from build123d import *

# Parameters (mm, degrees)
SKETCH1_W           = 127
SKETCH1_H           = 127
BOSS_EXTRUDE1_DEPTH = 127
SKETCH2_W           = 96.52
SKETCH2_H           = 96.52
CUT_EXTRUDE1_DEPTH  = 118.11
SKETCH3_W           = 101.6
SKETCH3_H           = 101.6
SKETCH3_W_2         = 96.52
SKETCH3_H_2         = 96.52
CUT_EXTRUDE2_DEPTH  = 6.35
SKETCH5_W           = 96.52
SKETCH5_H           = 105.41
CUT_EXTRUDE3_DEPTH  = 6.35
SKETCH6_W           = 109.22
SKETCH6_H           = 105.41
CUT_EXTRUDE4_DEPTH  = 6.35


with BuildPart() as part:
    # Sketch1 → Boss-Extrude1 (new body)
    with BuildSketch(Plane.XY):
        Rectangle(SKETCH1_W, SKETCH1_H)
    extrude(amount=BOSS_EXTRUDE1_DEPTH)

    # Sketch2 → Cut-Extrude1 (cut)
    with BuildSketch(Plane(origin=(0, 63.5, 0), x_dir=(1, 0, 0), z_dir=(0, 1, 0))):
        with Locations((0, -63.5)):
            Rectangle(SKETCH2_W, SKETCH2_H)
    extrude(amount=-CUT_EXTRUDE1_DEPTH, mode=Mode.SUBTRACT)

    # Sketch3 → Cut-Extrude2 (cut)
    with BuildSketch(Plane(origin=(0, 63.5, 0), x_dir=(1, 0, 0), z_dir=(0, 1, 0))):
        with Locations((0, -63.5)):
            Rectangle(SKETCH3_W, SKETCH3_H)
        with Locations((0, -63.5)):
            Rectangle(SKETCH3_W_2, SKETCH3_H_2, mode=Mode.SUBTRACT)
    extrude(amount=-CUT_EXTRUDE2_DEPTH, mode=Mode.SUBTRACT)

    # Sketch5 → Cut-Extrude3 (cut)
    with BuildSketch(Plane.XY.offset(15.24)):
        with Locations((0, -1.905)):
            Rectangle(SKETCH5_W, SKETCH5_H)
    cut_extrude3 = extrude(amount=-CUT_EXTRUDE3_DEPTH, mode=Mode.SUBTRACT)

    # Mirror1: Cut-Extrude3 across plane
    add(cut_extrude3.mirror(Plane(origin=(0, 0, 63.5), x_dir=(1, 0, 0), z_dir=(0, 0, -1))), mode=Mode.SUBTRACT)

    # Sketch6 → Cut-Extrude4 (cut)
    with BuildSketch(Plane.ZY.offset(-48.26)):
        with Locations((63.5, -1.905)):
            Rectangle(SKETCH6_W, SKETCH6_H)
    cut_extrude4 = extrude(amount=-CUT_EXTRUDE4_DEPTH, mode=Mode.SUBTRACT)

    # Mirror2: Cut-Extrude4 across plane
    add(cut_extrude4.mirror(Plane(origin=(0, 0, 0), x_dir=(0, 0, 1), z_dir=(1, 0, 0))), mode=Mode.SUBTRACT)


solid = part.part
Model file for the job. Use its own axes, mm. A direction names the side the tool comes from. Coordinates: 2 decimals unless noted, no trailing zeros. Write each loop counter-clockwise with the first axis right and the second up, starting at its lowest first coordinate (ties: lowest second). Pieces come first, ordered by that corner, then holes. Notation, with made-up numbers: (4, 78) -> (44, 78) arc R9 ccw to (44, 92) -> close; hole circle Ø10 at (-31.75, 28.25). An arc over 180 degrees is marked (long way). One line per item, written item: value. Start each with the question number.
1) Slice it at C-C on z = 93.5. Write the cut outline in (x, y).
2) Probe probe 1 along Y at (x, z) = (52.5, 93); probe 2 along X at (y, z) = (-3, 11); probe 3 along Z at (x, y) = (-53.5, 0). List the from-to ranges inside material, lowest first.
3) Slice it at B-B on x = -7. Write the cut outline in (y, z).
4) Slice it at A-A on y = -6. Write the cut outline in (x, z), then the cut area to 3 significant figures.
5) Which spindle directions (+Z, -Z, +X, -X, +Y, -Y) get a long thin tool onto all of the face, cutting with end or side? Do faces 1 (the face through (-63.5, -1, 63)), 2 (the face through (-49, 50.8, 63)), 3 (the face through (-1, 54, 15.24)). Say none if no direction does.
6) Pull direction Z, two halves, no side cores. Call faces 4 (the face through (-1, -63.5, 63)), 5 (the face through (-1, 1, 127)), 6 (the face through (-1, -1, 118.11)), 7 (the face through (-1, 1, 0)): +Z half, -Z half, draft (parallel to the pull), parting line (faces both ways), or undercut.
Answers follow:
1. outline: (-63.5, -63.5) -> (63.5, -63.5) -> (63.5, 63.5) -> (50.8, 63.5) -> (50.8, 57.15) -> (48.26, 57.15) -> (48.26, 50.8) -> (54.61, 50.8) -> (54.61, -54.61) -> (-54.61, -54.61) -> (-54.61, 50.8) -> (-48.26, 50.8) -> (-48.26, 57.15) -> (-50.8, 57.15) -> (-50.8, 63.5) -> (-63.5, 63.5) -> close
2. probe 1: -63.5 to -54.61, 50.8 to 63.5
2. probe 2: -63.5 to -54.61, 54.61 to 63.5
2. probe 3: 0 to 8.89, 118.11 to 127
3. outline: (-63.5, 0) -> (63.5, 0) -> (63.5, 12.7) -> (57.15, 12.7) -> (57.15, 15.24) -> (50.8, 15.24) -> (50.8, 8.89) -> (-54.61, 8.89) -> (-54.61, 118.11) -> (50.8, 118.11) -> (50.8, 111.76) -> (57.15, 111.76) -> (57.15, 114.3) -> (63.5, 114.3) -> (63.5, 127) -> (-63.5, 127) -> close
4. outline: (-63.5, 0) -> (63.5, 0) -> (63.5, 127) -> (-63.5, 127) -> close; hole (-54.61, 8.89) -> (54.61, 8.89) -> (54.61, 118.11) -> (-54.61, 118.11) -> close
4. area: 4,200 mm2
5. face 1: +Z, -Z, -X, +Y, -Y
5. face 2: none
5. face 3: +Y
6. face 4: draft
6. face 5: +Z half
6. face 6: undercut
6. face 7: -Z half
